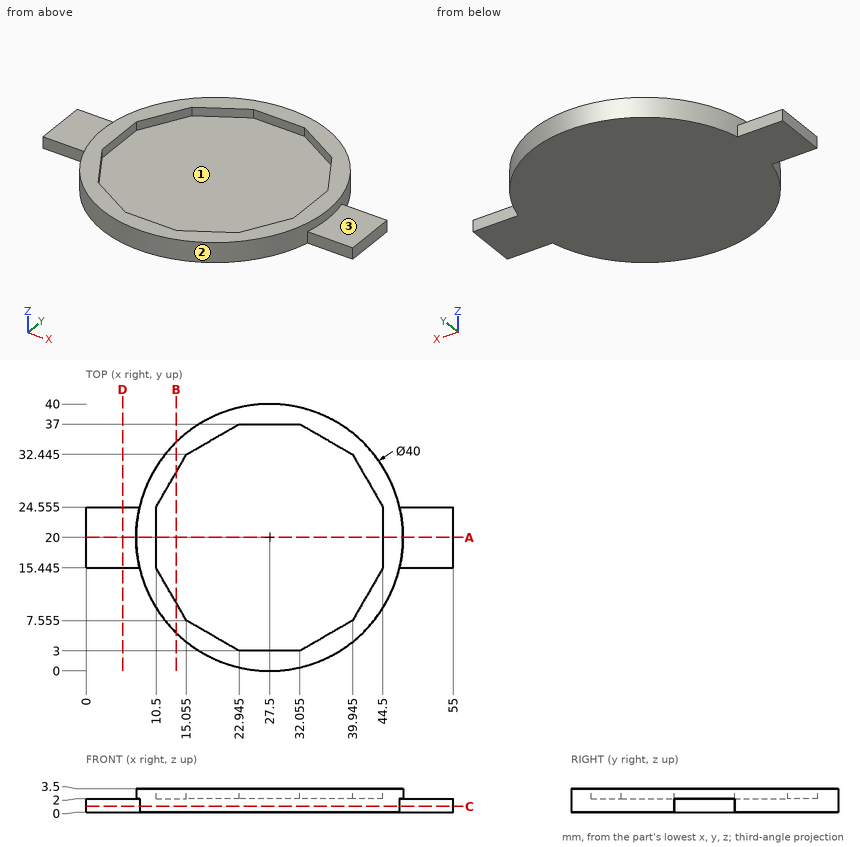
Can you work these out from the drawing? Everything is in mm from the part's minimum corner. Give positions to 0.01 mm unless a question says otherwise; leave off trailing zeros. Loops run counter-clockwise (first coordinate to the right, second up) from the corner with the lowest first, then second, coordinate; pieces in that order, holes last. Notation, with made-up numbers: (14.5, 42) - (29.5, 42) arc R26 ccw to (29.5, 57) - close; hole circle Ø1 at (19, 58.25). An arc over 180 degrees is marked (long way). Use one line per item in the form item = value.
1. Thinking about a two-plate mould opening in Y: for the marked faces 1, 2 and 3, which applies, released by +Y, released by -Y, zero draft, split by the parting line, or undercut?
Response values:
face_1 = undercut
face_2 = split by the parting line
face_3 = zero draft
2. I want a section at C-C (z = 0.9). Please give me the cut outline in (x, y) (1 decimal), and give its area (3 significant figures).
Response values:
outline = (0, 15.4) - (8, 15.4) arc R20 ccw to (47, 15.4) - (55, 15.4) - (55, 24.6) - (47, 24.6) arc R20 ccw to (8, 24.6) - (0, 24.6) - close
area = 1,400 mm²
3. I want a section at A-A (y = 20). Please give me the cut outline in (x, z).
Response values:
outline = (0, 0) - (55, 0) - (55, 2) - (47.5, 2) - (47.5, 3.5) - (44.5, 3.5) - (44.5, 2) - (10.5, 2) - (10.5, 3.5) - (7.5, 3.5) - (7.5, 2) - (0, 2) - close
4. I'm going to push flat-ended pins straight in: pin 1 Ø0.6 at (x, z) = (5, 1.5) entering from +Y (3 decimals); pin 2 Ø0.8 at (y, z) = (18.5, 2.5) entering from -X; pin 3 Ø0.8 at (x, z) = (29, 3) entering from -Y. Where does each tip first touch, or does it pass through?
Response values:
pin_1 = 24.555
pin_2 = 7.53
pin_3 = 0.03
5. I need wall thicknesses on probe 1 along Z at (x, y) = (32, 19); probe 2 along X at (y, z) = (34.5, 2.55) (1 decimal); probe 3 along Y at (x, z) = (17.5, 2.9). Which ranges of each line are inside material? Lowest first, please.
Response values:
probe_1 = 0 to 2
probe_2 = 13.7 to 18.6, 36.4 to 41.3
probe_3 = 2.68 to 6.14, 33.86 to 37.32
6. I want a section at B-B (x = 13.5). Please give me the cut outline in (y, z), and give its area (3 significant figures).
Response values:
outline = (5.72, 0) - (34.28, 0) - (34.28, 3.5) - (29.75, 3.5) - (29.75, 2) - (10.25, 2) - (10.25, 3.5) - (5.72, 3.5) - close
area = 70.7 mm²
7. I want a section at D-D (x = 5.5). Please give me the cut outline in (y, z) (3 decimals).
Response values:
outline = (15.445, 0) - (24.555, 0) - (24.555, 2) - (15.445, 2) - close
